```python
from build123d import *

# Parameters (mm, degrees)
SKETCH1_R           = 4
BOSS_EXTRUDE1_DEPTH = 5
BOSS_EXTRUDE2_DEPTH = 7
BOSS_EXTRUDE3_DEPTH = 16
SKETCH6_R           = 7
SKETCH6_R_2         = 4
BOSS_EXTRUDE4_DEPTH = 2.5
CUT_EXTRUDE1_DEPTH  = 4.4
CUT_EXTRUDE2_DEPTH  = 21.4
SKETCH8_R           = 2.25
CUT_EXTRUDE3_DEPTH  = 36.75
SKETCH9_R           = 4
CUT_EXTRUDE4_DEPTH  = 4


with BuildPart() as part:
    # Sketch1 → Boss-Extrude1 (new body)
    with BuildSketch(Plane(origin=(0, 0, 0), x_dir=(1, 0, 0), z_dir=(0, 1, 0))):
        Polygon((-4.25, 8.75), (18.75, 8.75), (23.75, 5.25), (23.75, -19.25), (15.75, -27), (-19.25, -27), (-19.25, -25), (-8.5, -18.25), (-2.25, -18.25), (-2.25, -10.25), (-9.25, -5.25), (-9.25, 3.75), align=None)
        Circle(SKETCH1_R, mode=Mode.SUBTRACT)
        with Locations((15.75, 0)):
            Circle(SKETCH1_R, mode=Mode.SUBTRACT)
    extrude(amount=BOSS_EXTRUDE1_DEPTH)

    # Sketch2 → Boss-Extrude2 (add)
    with BuildSketch(Plane.XZ):
        Polygon((23.75, 19.25), (23.75, -5.25), (20.25, -5.25), (20.25, 18.25), (-8.5, 18.25), (-14.87037037, 22.25), (20.653225806, 22.25), align=None)
    extrude(amount=BOSS_EXTRUDE2_DEPTH)

    # Sketch3 → Boss-Extrude3 (add)
    with BuildSketch(Plane.XZ):
        Polygon((-14.87037037, 22.25), (20.653225806, 22.25), (15.75, 27), (-19.25, 27), (-19.25, 25), align=None)
    extrude(amount=BOSS_EXTRUDE3_DEPTH)

    # Sketch6 → Boss-Extrude4 (add)
    with BuildSketch(Plane.XZ):
        with Locations((15.75, 0)):
            Circle(SKETCH6_R)
        with Locations((15.75, 0)):
            Circle(SKETCH6_R_2, mode=Mode.SUBTRACT)
    extrude(amount=BOSS_EXTRUDE4_DEPTH)

    # Sketch4 → Cut-Extrude1 (cut)
    with BuildSketch(Plane.XZ):
        with BuildLine():
            Line((5.883782294, -1), (12.395898034, -1))
            ThreePointArc((12.395898034, -1), (12.25, 0), (12.395898034, 1))
            Line((12.395898034, 1), (5.883782294, 1))
            ThreePointArc((5.883782294, 1), (-5.968156673, 0), (5.883782294, -1))
        make_face()
    extrude(amount=-CUT_EXTRUDE1_DEPTH, mode=Mode.SUBTRACT)

    # Sketch7 → Cut-Extrude2 (cut, through all)
    with BuildSketch(Plane.XZ.offset(-4.4)):
        with BuildLine():
            Line((5.883782294, -1), (11.877016654, -1))
            ThreePointArc((11.877016654, -1), (11.75, 0), (11.877016654, 1))
            Line((11.877016654, 1), (5.883782294, 1))
            ThreePointArc((5.883782294, 1), (-5.968156673, 0), (5.883782294, -1))
        make_face()
    extrude(amount=CUT_EXTRUDE2_DEPTH, mode=Mode.SUBTRACT)

    # Sketch8 → Cut-Extrude3 (cut, through all)
    with BuildSketch(Plane.XY.offset(27)):
        with Locations((10.75, -5)):
            Circle(SKETCH8_R)
        with Locations((-9.25, -5)):
            Circle(SKETCH8_R)
    extrude(amount=-CUT_EXTRUDE3_DEPTH, mode=Mode.SUBTRACT)

    # Sketch9 → Cut-Extrude4 (cut)
    with BuildSketch(Plane(origin=(0, 0, 18.25), x_dir=(-1, 0, 0), z_dir=(0, 0, -1))):
        with Locations((-10.75, -5)):
            Circle(SKETCH9_R)
        with Locations((9.25, -5)):
            Circle(SKETCH9_R)
    extrude(amount=-CUT_EXTRUDE4_DEPTH, mode=Mode.SUBTRACT)


solid = part.part
```
The model under review builds one solid part; all positions refer to its coordinate system, in mm. A direction names the side the tool comes from. Round coordinates to 2 decimals unless told otherwise and drop trailing zeros. Loops run counter-clockwise (first coordinate to the right, second up) from the corner with the lowest first, then second, coordinate; pieces in that order, holes last. Notation, with made-up numbers: M 16.25,-21.5 L 43.25,-21.5 A16 ccw 43.25,-0.5 Z; hole C -3,79.25 d1. An arc over 180 degrees is marked long. Write item = value, one per line.
Item 1: Take a section at B-B on x = 0. Write out the cut boundary in (y, z), then the cut area to 3 significant figures.
Return value:
outline = M -16,22.25 L -7,22.25 L -7,18.25 L 0,18.25 L 0,5.97 L 4.4,5.97 L 4.4,4 L 5,4 L 5,27 L -16,27 Z; M 0,-8.75 L 5,-8.75 L 5,-4 L 4.4,-4 L 4.4,-5.97 L 0,-5.97 Z
area = 225 mm2
Item 2: For line 1 (Y direction, x = 10.75, z = 24.2); line 2 (Z direction, x = 8, y = 2.5); line 3 (X direction, y = 1.65, z = 0), list the stretches that pass through material, from the lowest coordinate up. Write a range as [from, to].
Return value:
line_1 = [-16, -7.25], [-2.75, 5]
line_2 = [-8.75, -1], [1, 27]
line_3 = [-9.25, -5.97], [19.75, 23.75]
Item 3: The part is to be moulded in two halves that separate along X. For faces 6 (the flat face through (21, -7, 12)), 7 (the flat face through (9, 2, 1)), 8 (the flat face through (-9.25, 2, 1)), say which applies: released by +X, released by -X, zero draft, split by the parting line, or undercut.
Return value:
face_6 = zero draft
face_7 = undercut
face_8 = released by -X
Item 4: Machinability: for faces 1 (the cylindrical face through (13.236, -1.232, -6.533)), 2 (the flat face through (-14, -7, 22)), 3 (the flat face through (0, -16, 25)), 4 (the cylindrical face through (10.63, -1, 20.22)), 5 (the cylindrical face through (-7.56, -1.374, 20.666)), which of the approach directions +Z, -Z, +X, -X, +Y, -Y give a long, thin tool a straight path to every point of the face, cutting with its end or side? Answer none if there is none.
Return value:
face_1 = -Z, -Y
face_2 = -Z, +X, -X, -Y
face_3 = +Z, -Z, +X, -X, -Y
face_4 = none
face_5 = -Z
Item 5: Take a section at C-C on y = -5. Write out the cut boundary in (x, z).
Return value:
outline = M -19.25,25 L -13.25,21.23 L -13.25,22.25 L -11.5,22.25 L -11.5,27 L -19.25,27 Z; M -7,22.25 L -5.25,22.25 L -5.25,18.25 L 6.75,18.25 L 6.75,22.25 L 8.5,22.25 L 8.5,27 L -7,27 Z; M 13,22.25 L 14.75,22.25 L 14.75,18.25 L 20.25,18.25 L 20.25,-5.25 L 23.75,-5.25 L 23.75,19.25 L 15.75,27 L 13,27 Z
Item 6: Take a section at A-A on z = 0. Write out the cut boundary in (x, y), then the cut area to 3 significant figures.
Return value:
outline = M -9.25,0 L -5.97,0 L -5.97,4.4 L -4,4.4 L -4,5 L -9.25,5 Z; M 4,4.4 L 11.75,4.4 L 11.75,5 L 4,5 Z; M 19.75,-2.5 L 20.25,-2.5 L 20.25,-7 L 23.75,-7 L 23.75,5 L 19.75,5 Z
area = 68.0 mm2
Item 7: Insertion check: P1, Ø2, axis at y = -4.5, z = 11.5, coming from the -X side; P2, Ø4, axis at y = 3, z = 1, coming from the -X side; P3, Ø12, axis at x = 17, y = -3.5, coming from the -Z side; P4, Ø2.5, axis at y = 3, z = 15.5, coming from the -X side. Each pin has a flat end and moves straight along its axis. Give the tip position at first contact, or say it passes through.
Return value:
P1 = 20.25
P2 = -9.25
P3 = -8.75
P4 = -2.25
Item 8: Take a section at D-D on z = 9. Write out the cut boundary in (x, y), then the cut area to 3 significant figures.
Return value:
outline = M -4,0 L 20.25,0 L 20.25,-7 L 23.75,-7 L 23.75,5 L -4,5 Z
area = 163 mm2
